from build123d import *

# Parameters (mm, degrees)
BOSS_EXTRUDE1_DEPTH     = 50
CUT_EXTRUDE2_DEPTH      = 53.528563658
CUT_EXTRUDE2_DEPTH_BACK = 53.528563658
SKETCH7_R               = 1.5


with BuildPart() as part:
    # Sketch1 → Boss-Extrude1 (new body)
    with BuildSketch(Plane.XY):
        with BuildLine():
            Line((-7, 12.698425099), (-7, 8.614522622))
            ThreePointArc((-7, 8.614522622), (0, 11.1), (7, 8.614522622))
            Line((7, 8.614522622), (7, 12.698425099))
            ThreePointArc((7, 12.698425099), (0, 14.5), (-7, 12.698425099))
        make_face()
    extrude(amount=BOSS_EXTRUDE1_DEPTH)

    # Sketch7 → Cut-Extrude2 (cut, two sides: drawn at the far end of the back side and taken through both)
    with BuildSketch(Plane(origin=(0, 0, 0), x_dir=(1, 0, 0), z_dir=(0, 1, 0)).offset(-CUT_EXTRUDE2_DEPTH_BACK)):
        with Locations(Location((0, -8, 0), (0, 0, 90))):
            Circle(SKETCH7_R)
        with Locations(Location((0, -42, 0), (0, 0, 90))):
            Circle(SKETCH7_R)
    extrude(amount=CUT_EXTRUDE2_DEPTH + CUT_EXTRUDE2_DEPTH_BACK, mode=Mode.SUBTRACT)


solid = part.part
Read the model definition and answer for the solid it produces. Units are mm, in the model's axes. Coordinates: 2 decimals unless noted, no trailing zeros. Write each loop counter-clockwise with the first axis right and the second up, starting at its lowest first coordinate (ties: lowest second). Pieces come first, ordered by that corner, then holes. Notation, with made-up numbers: (-22, 49.5) - (1, 49.5) arc R20 ccw to (1, 60.5) - close; hole circle Ø6 at (77, 35.25). An arc over 180 degrees is marked (long way). One line per question, with ' | ' between items.
Q1. Find section B-B, the plane y = 9.1. Write down the section's boundary in (x, z).
Result set:
outline: (-7, 0) - (-6.36, 0) - (-6.36, 50) - (-7, 50) - close; (6.36, 0) - (7, 0) - (7, 50) - (6.36, 50) - close
Q2. Find section D-D, the plane y = 11.55. Write down the section's boundary in (x, z), plus the area to 3 significant figures.
Result set:
outline: (-7, 0) - (7, 0) - (7, 50) - (-7, 50) - close; hole circle Ø3 at (0, 8); hole circle Ø3 at (0, 42) | area: 686 mm^2
Q3. Find section A-A, the plane x = 0. Write down the section's boundary in (y, z).
Result set:
outline: (11.1, 0) - (14.5, 0) - (14.5, 6.5) - (11.1, 6.5) - close; (11.1, 9.5) - (14.5, 9.5) - (14.5, 40.5) - (11.1, 40.5) - close; (11.1, 43.5) - (14.5, 43.5) - (14.5, 50) - (11.1, 50) - close
Q4. Determine the mould class of faces 1 (the cylindrical face through (-0.1, 11.1, 24.6)), 2 (the flat face through (7, 11, 25)), 3 (the flat face through (0, 12, 50)) for opening direction X: +X half, -X half, draft (parallel to the pull), parting line (faces both ways), or undercut.
Result set:
face 1: undercut | face 2: +X half | face 3: draft
Q5. Each of these flat-tipped pins is pushed along its axis until it touches: P1, Ø1.5, axis at x = -3.5, y = 10, coming from the -Z side; P2, Ø6, axis at x = -3, z = 9, coming from the -Y side; P3, Ø3, axis at x = -3.5, z = 44, coming from the +Y side. Where does it stop, or does it pass through?
Result set:
P1: z = 0 | P2: y = 9.34 | P3: y = 14.36
Q6. Consider L1, parallel to X at y = 12.1, z = 8; L2, parallel to X at y = 13.4, z = 8; L3, parallel to Y at x = -0.5, z = 30.5. Determine where each line is inside the solid, lowest interval first. Write a range as [from, to].
Result set:
L1: [-7, -1.5], [1.5, 7] | L2: [-5.54, -1.5], [1.5, 5.54] | L3: [11.09, 14.49]
Q7. Find section C-C, the plane z = 8. Write down the section's boundary in (x, y).
Result set:
outline: (-7, 8.61) arc R11.1 cw to (-1.5, 11) - (-1.5, 14.42) arc R14.5 ccw to (-7, 12.7) - close; (1.5, 11) arc R11.1 cw to (7, 8.61) - (7, 12.7) arc R14.5 ccw to (1.5, 14.42) - close
